Can you work these out from the drawing? Everything is in mm from the part's minimum corner. Coordinates: 2 decimals unless noted, no trailing zeros. Loops run counter-clockwise (first coordinate to the right, second up) from the corner with the lowest first, then second, coordinate; pieces in that order, holes last.
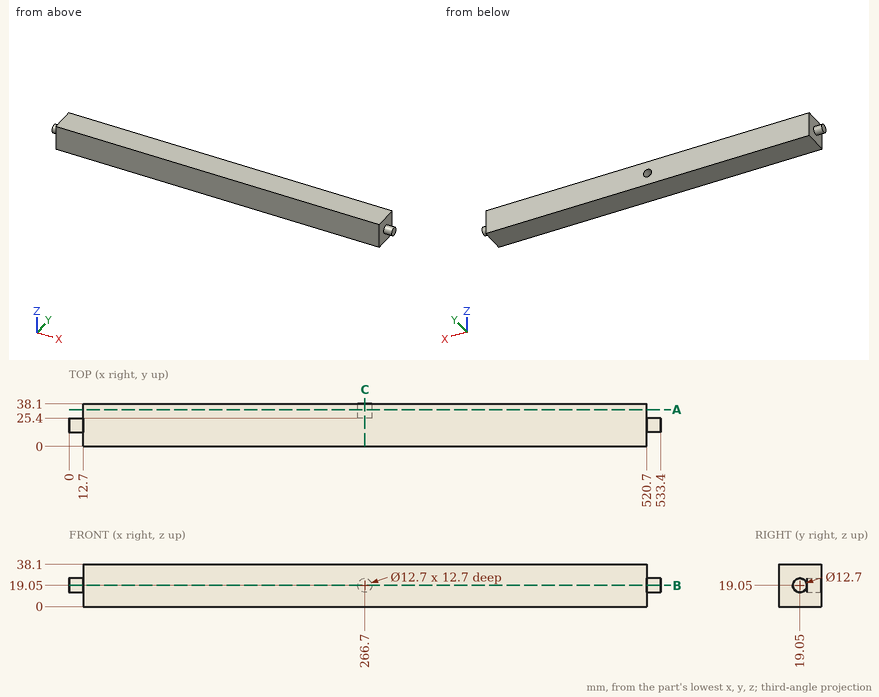
(1) I need wall thicknesses on probe 1 along Z at (x, y) = (266, 33); probe 2 along X at (y, z) = (29, 19.05); probe 3 along X at (y, z) = (27, 7.5). Which ranges of each line are inside material? Lowest first, please.
Answers:
probe 1: z = 0 to 12.74, 25.36 to 38.1
probe 2: x = 12.7 to 260.35, 273.05 to 520.7
probe 3: x = 12.7 to 520.7
(2) For pin 1 (2 mm diameter, centred on y = 32.5, z = 16, fed in from -X); pin 2 (8 mm diameter, centred on y = 5.5, z = 15, fed in from +X), each with a flat end and sliding along its axis, tell me the tip position at first contact or that it passes through.
Answers:
pin 1: stops at x = 12.7
pin 2: stops at x = 520.7
(3) Imagine slicing it at B-B, the plane z = 19.05. Write out the boundary of the cut face in (x, y).
Answers:
outline: (0, 12.7) - (12.7, 12.7) - (12.7, 0) - (520.7, 0) - (520.7, 12.7) - (533.4, 12.7) - (533.4, 25.4) - (520.7, 25.4) - (520.7, 38.1) - (273.05, 38.1) - (273.05, 25.4) - (260.35, 25.4) - (260.35, 38.1) - (12.7, 38.1) - (12.7, 25.4) - (0, 25.4) - close
(4) Imagine slicing it at C-C, the plane x = 266.7. Write out the boundary of the cut face in (y, z), and give its area (3 significant figures).
Answers:
outline: (0, 0) - (38.1, 0) - (38.1, 12.7) - (25.4, 12.7) - (25.4, 25.4) - (38.1, 25.4) - (38.1, 38.1) - (0, 38.1) - close
area: 1,290 mm2
(5) Imagine slicing it at A-A, the plane y = 33. Write out the boundary of the cut face in (x, z).
Answers:
outline: (12.7, 0) - (520.7, 0) - (520.7, 38.1) - (12.7, 38.1) - close; hole circle Ø12.7 at (266.7, 19.05)
